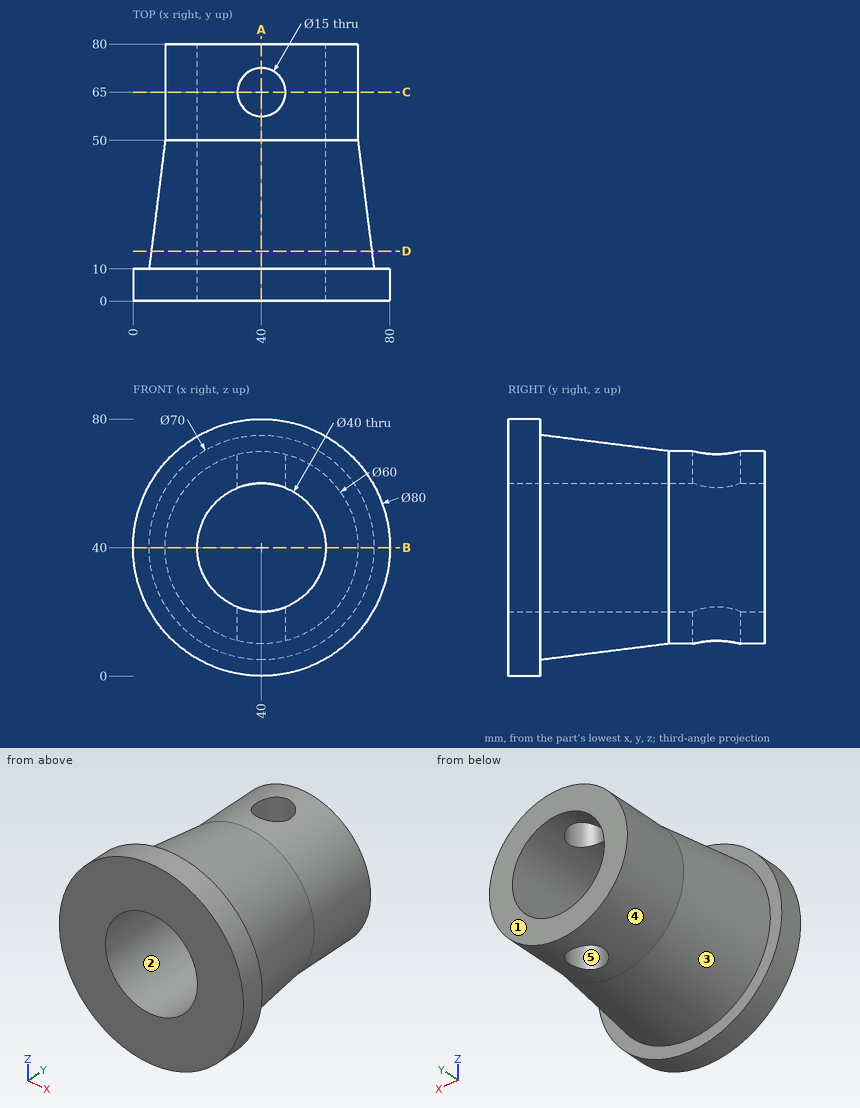
Input: dimensioned drawing with shaded views. Units: mm. Origin: part minimum x, y, z. A direction names the side the tool comes from. Round coordinates to 2 decimals unless told otherwise and drop trailing zeros. Loops run counter-clockwise (first coordinate to the right, second up) from the corner with the lowest first, then second, coordinate; pieces in that order, holes last.
1) Section query A-A on x = 40. Return the cut outline in (y, z), plus the area to 3 significant figures.
Ans:
outline: (0, 0) - (10, 0) - (10, 5) - (50, 10) - (57.5, 10) - (57.5, 20) - (0, 20) - close; (0, 60) - (57.5, 60) - (57.5, 70) - (50, 70) - (10, 75) - (10, 80) - (0, 80) - close; (72.5, 10) - (80, 10) - (80, 20) - (72.5, 20) - close; (72.5, 60) - (80, 60) - (80, 70) - (72.5, 70) - close
area: 1,700 mm2
2) Pin query (flat end, axial travel): pin 1 (10 mm diameter, centred on x = 32.5, y = 18, fed in from -Z); pin 2 (4 mm diameter, centred on x = 50, y = 47, fed in from -Z); pin 3 (1.5 mm diameter, centred on x = 65, y = 58.5, fed in from -Z). Return the tip coordinate at first contact, or that it passes through.
Ans:
pin 1: stops at z = 5.79
pin 2: stops at z = 10.64
pin 3: stops at z = 22.34
3) Section query C-C on y = 65. Return the cut outline in (x, z).
Ans:
outline: (32.5, 10.95) - (32.5, 21.46) arc R20 cw to (32.5, 58.54) - (32.5, 69.05) arc R30 ccw to start; (47.5, 10.95) arc R30 ccw to (47.5, 69.05) - (47.5, 58.54) arc R20 cw to (47.5, 21.46) - close
4) Section query D-D on y = 15.5. Return the cut outline in (x, z) (1 decimal).
Ans:
outline: circle Ø68.6 at (40, 40); hole circle Ø40 at (40, 40)
5) Section query B-B on z = 40. Return the cut outline in (x, y), plus the area to 3 significant figures.
Ans:
outline: (0, 0) - (20, 0) - (20, 80) - (10, 80) - (10, 50) - (5, 10) - (0, 10) - close; (60, 0) - (80, 0) - (80, 10) - (75, 10) - (70, 50) - (70, 80) - (60, 80) - close
area: 2,000 mm2
6) Material intervals for line 1 (Y direction, x = 40, z = 61.5); line 2 (X direction, y = 54, z = 40), sorted ascending.
Ans:
line 1: y = 0 to 57.5, 72.5 to 80
line 2: x = 10 to 20, 60 to 70
7) Pull-direction query (X, two-part tool) for the marked faces 1, 2 and 3; classes: released by +X, released by -X, zero draft, split by the parting line, or undercut.
Ans:
face 1: zero draft
face 2: undercut
face 3: split by the parting line
8) Set-up query: the marked faces 4 and 5. Return all of +Z, -Z, +X, -X, +Y, -Y with unobstructed straight access to the full face (end or side cutting, diameter ignored); none if empty.
Ans:
face 4: +Y
face 5: +Z, -Z
